Work out the finished part from the listing and answer in its coordinate system (mm). A direction names the side the tool comes from. Round coordinates to 2 decimals unless told otherwise and drop trailing zeros. Write each loop counter-clockwise with the first axis right and the second up, starting at its lowest first coordinate (ties: lowest second). Pieces come first, ordered by that corner, then holes. Notation, with made-up numbers: (6, 68) - (31, 68) arc R23 cw to (31, 104) - close; hole circle Ø1 at (49.5, 15.25). An arc over 180 degrees is marked (long way). Answer as a JSON object with one key per item and string values.
```python
from build123d import *

# Parameters (mm, degrees)
F1_DEPTH = 10
F0_R     = 14.45
F2_DEPTH = 1.5875
F3_R     = 1.6
F4_DEPTH = 6.35
F5_DEPTH = 2
F6_DEPTH = 2
F7_DEPTH = 10
F8_DEPTH = 2.5


with BuildPart() as f1:
    # F0 (on Front) → F1 (new body)
    with BuildSketch(Plane.XZ):
        with BuildLine():
            Line((-60.452, 3.175), (-60.452, 0))
            Line((-60.452, 0), (-15.875, 0))
            Line((-15.875, 0), (15.85, 0))
            Line((15.85, 0), (60.452, 0))
            Line((60.452, 0), (60.452, 3.175))
            Line((60.452, 3.175), (31.025, 3.175))
            Line((31.025, 3.175), (19.025, 3.175))
            Line((19.025, 3.175), (19.025, 15.175))
            Line((19.025, 15.175), (19.025, 17.53616))
            Line((19.025, 17.53616), (19.025, 18.46384))
            ThreePointArc((19.025, 18.46384), (-0.231937, 37.02924), (-19.030653, 18))
            Line((-19.030653, 18), (-19.030653, 15.175))
            Line((-19.030653, 15.175), (-19.030653, 3.175))
            Line((-19.030653, 3.175), (-31.030653, 3.175))
            Line((-31.030653, 3.175), (-60.452, 3.175))
        make_face()
        with BuildLine():
            ThreePointArc((-16.05, 18), (-1.266886, 33.999922), (15.85, 20.525866))
            ThreePointArc((15.85, 20.525866), (15.999922, 19.266886), (16.05, 18))
            ThreePointArc((16.05, 18), (0, 1.95), (-16.05, 18))
        make_face(mode=Mode.SUBTRACT)
    extrude(amount=F1_DEPTH)

    # F0 (on Front) → F2 (join)
    with BuildSketch(Plane.XZ):
        with BuildLine():
            ThreePointArc((16.05, 18), (15.999922, 19.266886), (15.85, 20.525866))
            ThreePointArc((15.85, 20.525866), (-1.266886, 33.999922), (-16.05, 18))
            ThreePointArc((-16.05, 18), (0, 1.95), (16.05, 18))
        make_face()
        with Locations((0, 18)):
            Circle(F0_R, mode=Mode.SUBTRACT)
    extrude(amount=F2_DEPTH)

    # F3 (on face) → F4 (cut)
    with BuildSketch(Plane(origin=(0, 0, 0), x_dir=(1, 0, 0), z_dir=(0, 0, -1))):
        with Locations((-54.263, 6.35)):
            Circle(F3_R)
        with Locations((54.737, 6.35)):
            Circle(F3_R)
    extrude(amount=-F4_DEPTH, mode=Mode.SUBTRACT)

    # F0 (on Front) → F5 (join)
    with BuildSketch(Plane.XZ):
        with BuildLine():
            ThreePointArc((16.05, 18), (15.999922, 19.266886), (15.85, 20.525866))
            ThreePointArc((15.85, 20.525866), (-1.266886, 33.999922), (-16.05, 18))
            ThreePointArc((-16.05, 18), (0, 1.95), (16.05, 18))
        make_face()
        with Locations((0, 18)):
            Circle(F0_R, mode=Mode.SUBTRACT)
    extrude(amount=F5_DEPTH)

    # F0 (on Front) → F6 (join)
    with BuildSketch(Plane.XZ):
        Polygon((31.025, 3.175), (60.452, 3.175), (19.025, 17.53616), (19.025, 15.175), align=None)
        Polygon((-19.030653, 18), (-60.452, 3.175), (-31.030653, 3.175), (-19.030653, 15.175), align=None)
    extrude(amount=F6_DEPTH)

    # F0 (on Front) → F7 (join)
    with BuildSketch(Plane.XZ):
        Polygon((19.025, 3.175), (31.025, 3.175), (19.025, 15.175), align=None)
        Polygon((-19.030653, 15.175), (-31.030653, 3.175), (-19.030653, 3.175), align=None)
    extrude(amount=F7_DEPTH)

    # F0 (on Front) → F8 (join)
    with BuildSketch(Plane.XZ):
        Polygon((31.025, 3.175), (60.452, 3.175), (19.025, 17.53616), (19.025, 15.175), align=None)
        Polygon((-19.030653, 18), (-60.452, 3.175), (-31.030653, 3.175), (-19.030653, 15.175), align=None)
    extrude(amount=F8_DEPTH)


solid = f1.part
```
Item 1: A cutting plane is placed at D-D (z = 26). Write down the section's boundary in (x, y), and give its area (3 significant figures).
Results found:
{"outline": "(-17.27, -10) - (-13.91, -10) - (-13.91, -2) - (-12.03, -2) - (-12.03, 0) - (-17.27, 0) - close; (12.03, -2) - (13.91, -2) - (13.91, -10) - (17.27, -10) - (17.27, 0) - (12.03, 0) - close", "area": "74.6 mm²"}
Item 2: A cutting plane is placed at C-C (z = 13). Write down the section's boundary in (x, y).
Results found:
{"outline": "(-33, -2.5) - (-21.21, -2.5) - (-21.21, -10) - (-15.25, -10) - (-15.25, -2) - (-13.56, -2) - (-13.56, 0) - (-33, 0) - close; (13.56, -2) - (15.25, -2) - (15.25, -10) - (21.2, -10) - (21.2, -2.5) - (32.11, -2.5) - (32.11, 0) - (13.56, 0) - close"}
Item 3: For faces 4 (the flat face through (25.1, -6.2, 9.1)), 5 (the flat face through (-12, -2, 26.4)), 6 (the flat face through (-46, -6, 3.175)), determine the directions among +Z, -Z, +X, -X, +Y, -Y from which every point of the face is accessible in a straight line to the end or side of a thin tool.
Results found:
{"face 4": "+Z, +X, -Y", "face 5": "-Y", "face 6": "+Z, -X, -Y"}
Item 4: Consider line 1 along X through (y, z) = (-6.35, 1.65); line 2 along Z through (x, y) = (0, -0.85); line 3 along Z through (x, y) = (-49, -8.75) (3 decimals). Determine where each line is inside the solid, lowest interval first.
Results found:
{"line 1": "-60.45 to -55.86, -52.66 to 53.14, 56.34 to 60.45", "line 2": "0 to 3.55, 32.45 to 37.03", "line 3": "0 to 3.175"}
Item 5: Determine the mould class of faces 1 (the flat face through (-35, -2.5, 8)), 2 (the cylindrical face through (7.768, -0.986, 30.184)), 3 (the flat face through (-24.947, -6.198, 9.259)) for opening direction Z: pulls with the +Z half, pulls with the -Z half, needs draft (parallel to the pull), parting line crosses it, or undercut.
Results found:
{"face 1": "needs draft", "face 2": "undercut", "face 3": "pulls with the +Z half"}
Item 6: Each of these flat-tipped pins is pushed along its axis until it touches: P1, Ø2, axis at y = -4.5, z = 9.5, coming from the -X side; P2, Ø3, axis at y = -5, z = 17, coming from the -X side; P3, Ø1.5, axis at x = -15.5, z = 32, coming from the -Y side; P4, Ø5, axis at y = -2.5, z = 24.5, coming from the +X side. Where does it stop, or does it pass through?
Results found:
{"P1": "x = -25.71", "P2": "x = -19.03", "P3": "through", "P4": "x = 18.61"}
Item 7: A cutting plane is placed at B-B (x = 0). Write down the section's boundary in (y, z), and give its area (3 significant figures).
Results found:
{"outline": "(-10, 0) - (0, 0) - (0, 3.55) - (-2, 3.55) - (-2, 1.95) - (-10, 1.95) - close; (-10, 34.05) - (-2, 34.05) - (-2, 32.45) - (0, 32.45) - (0, 37.03) - (-10, 37.03) - close", "area": "55.7 mm²"}
Item 8: A cutting plane is placed at A-A (y = -6.35). Write down the section's boundary in (x, z) (3 decimals).
Results found:
{"outline": "(-60.452, 0) - (-55.863, 0) - (-55.863, 3.175) - (-60.452, 3.175) - close; (-52.663, 0) - (53.137, 0) - (53.137, 3.175) - (31.025, 3.175) - (19.025, 15.175) - (19.025, 18.464) arc R19.031 ccw to (-19.031, 18) - (-19.031, 15.175) - (-31.031, 3.175) - (-52.663, 3.175) - close; (56.337, 0) - (60.452, 0) - (60.452, 3.175) - (56.337, 3.175) - close; hole (15.85, 20.526) arc R16.05 ccw (long way) to (16.05, 18) arc R16.05 ccw to start"}
